from build123d import *

# Parameters (mm, degrees)
EXTRUDE1_DEPTH            = 18.7198
SKETCH13_W                = 30.336118919
SKETCH13_H                = 26.43936277
EXTRUDE2_DEPTH            = 40.057833358
F_6_32_TAPPED_HOLE2_D     = 2.7051
EXTRUDE3_DEPTH            = 40.057833358
F_6_32_TAPPED_HOLE1_D     = 2.7051
F_8_32_TAPPED_HOLE5_D     = 3.4544
F_8_32_TAPPED_HOLE5_DEPTH = 19.05
F_8_32_TAPPED_HOLE5_TIP   = 1.037806461
SKETCH22_W                = 9.398
SKETCH22_H                = 21.690053411
EXTRUDE4_DEPTH            = 33.232321948
CHAMFER1_SIZE             = 5.588


with BuildPart() as part:
    # Sketch1 → Extrude1 (new body)
    with BuildSketch(Plane.XY):
        with BuildLine():
            Line((0, 0), (0, -13.17458008))
            Line((0, -13.17458008), (15.324208221, -28.498788301))
            ThreePointArc((15.324208221, -28.498788301), (19.05, -6.58729004), (15.324208221, 15.324208221))
            Line((15.324208221, 15.324208221), (0, 15.324208221))
            Line((0, 15.324208221), (0, 0))
        make_face()
    extrude(amount=EXTRUDE1_DEPTH)

    # Sketch13 → Extrude2 (cut, through all)
    with BuildSketch(Plane.XY.offset(18.7198)):
        with Locations((15.16805946, 17.825101305)):
            Rectangle(SKETCH13_W, SKETCH13_H)
    extrude(amount=-EXTRUDE2_DEPTH, mode=Mode.SUBTRACT)

    # #6-32 Tapped Hole2 (through all)
    with Locations(Plane.XY.offset(18.7198)):
        with Locations((13.6525, -1.50729004)):
            Hole(F_6_32_TAPPED_HOLE2_D / 2)

    # Sketch14 → Extrude3 (cut, through all)
    with BuildSketch(Plane.XY.offset(18.7198)):
        Polygon((0.684709755, -13.859289835), (7.276217748, -7.267781842), (18.052525094, -18.044089188), (21.915716214, -21.907280308), (15.324208221, -28.498788301), align=None)
    extrude(amount=-EXTRUDE3_DEPTH, mode=Mode.SUBTRACT)

    # #6-32 Tapped Hole1 (through all)
    with Locations(Plane(origin=(12.651735758, -12.643299852, 14.4399), x_dir=(-0.707106781187, 0.707106781187, 0), z_dir=(-0.707106781187, -0.707106781187, 0))):
        with Locations((0, 0), (0, 10.16)):
            Hole(F_6_32_TAPPED_HOLE1_D / 2)

    # #8-32 Tapped Hole5
    with Locations(Plane.ZY):
        with Locations((9.3599, -6.58729004)):
            Hole(F_8_32_TAPPED_HOLE5_D / 2, depth=F_8_32_TAPPED_HOLE5_DEPTH)
            with Locations((0, 0, -(F_8_32_TAPPED_HOLE5_DEPTH + F_8_32_TAPPED_HOLE5_TIP / 2))):  # 118° drill point
                Cone(0, F_8_32_TAPPED_HOLE5_D / 2, F_8_32_TAPPED_HOLE5_TIP, mode=Mode.SUBTRACT)

    # Sketch22 → Extrude4 (cut, through all)
    with BuildSketch(Plane.XY.offset(18.7198)):
        with Locations((4.699, -6.239606786)):
            Rectangle(SKETCH22_W, SKETCH22_H)
    extrude(amount=-EXTRUDE4_DEPTH, mode=Mode.SUBTRACT)

    # Chamfer1
    chamfer1_edges = [part.edges().sort_by_distance(p)[0] for p in [
        (9.398, 4.60541992, 9.3599),
    ]]
    chamfer(chamfer1_edges, length=CHAMFER1_SIZE)


solid = part.part
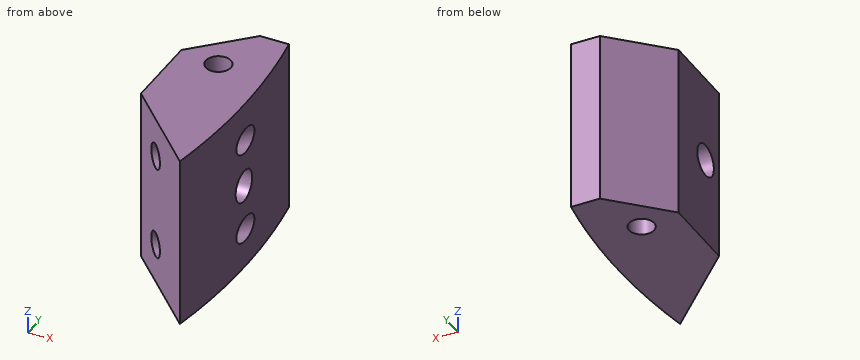
The model under review builds one solid part; all positions refer to its coordinate system, in mm. Give positions to 0.01 mm unless a question says otherwise; leave off trailing zeros. Order: outer loops, then holes, each group sorted by start corner. A loop starts at its lowest first (then second) coordinate and runs counter-clockwise, first axis right, second up. Notation, with made-up numbers: (29.25, 30) -> (50.25, 30) arc R12 cw to (50.25, 35) -> close; hole circle Ø4 at (56, 41.5). An arc over 180 degrees is marked (long way). Write item = value, one per line. Start each with the question number.
(1) For L1, parallel to Z at x = 17.25, y = -8; L2, parallel to Y at x = 18, z = 4; L3, parallel to Z at x = 14, y = -9.5, list the stretches that pass through material, from the lowest coordinate up. Write a range as from..to.
(2) Take a section at C-C (z = 14). Write out the cut boundary in (x, y).
(3) Take a section at D-D (z = 1). Write out the cut boundary in (x, y), plus the area to 3 significant figures.
(4) For pin 1 Ø1.6 at (x, y) = (13.65, -1.51) entering from -Z; pin 2 Ø4 at (y, z) = (-6.59, 9.36) entering from -X; pin 3 Ø1 at (x, z) = (12.5, 5) entering from +Y; pin 4 Ø1.5 at (x, z) = (14.5, 15.5) entering from -Y, all flat-tipped, find the tip position at first contact; note any pin that passes through.
(5) Take a section at A-A (z = 3.5). Write out the cut boundary in (x, y), plus the area to 3 significant figures.
(6) Take a section at B-B (x = 11.25). Write out the cut boundary in (y, z), plus the area to 3 significant figures.
Returned:
q1.L1 = 0..2.93, 5.63..8.37, 10.35..13.09, 15.79..18.72
q1.L2 = -17.99..-9.17, -5.42..4.61
q1.L3 = 0..3.81, 4.75..13.97, 14.91..18.72
q2.outline = (9.4, -9.39) -> (11.75, -11.74) -> (19.02, -4.47) arc R66.29 ccw to (18.1, 4.61) -> (14.99, 4.61) -> (9.4, -0.98) -> close; (13.56, -13.55) -> (18.05, -18.04) arc R66.29 ccw to (19.03, -8.07) -> close; hole circle Ø2.71 at (13.65, -1.51)
q3.outline = (9.4, -9.39) -> (18.05, -18.04) arc R66.29 ccw to (18.1, 4.61) -> (14.99, 4.61) -> (9.4, -0.98) -> close; hole circle Ø2.71 at (13.65, -1.51)
q3.area = 152 mm²
q4.pin_1 = through
q4.pin_2 = 9.4
q4.pin_3 = 2.62
q4.pin_4 = -15.24
q5.outline = (9.4, -9.39) -> (11.87, -11.86) -> (19.02, -4.71) arc R66.29 ccw to (18.1, 4.61) -> (14.99, 4.61) -> (9.4, -0.98) -> close; (13.43, -13.42) -> (18.05, -18.04) arc R66.29 ccw to (19.04, -7.82) -> close; hole circle Ø2.71 at (13.65, -1.51)
q5.area = 132 mm²
q6.outline = (-11.24, 0) -> (0.87, 0) -> (0.87, 18.72) -> (-11.24, 18.72) -> close; hole circle Ø3.45 at (-6.59, 9.36)
q6.area = 217 mm²
